The listing builds one solid part. Answer for the finished solid, in the listing's coordinates (mm). A direction names the side the tool comes from. Give positions to 0.01 mm unless a question says otherwise; leave off trailing zeros. Order: outer loops, then holes, each group sorted by start corner. A loop starts at its lowest first (then second) coordinate and runs counter-clockwise, first axis right, second up. Notation, with made-up numbers: (75.25, -15) -> (106.25, -15) arc R18 cw to (106.25, 17) -> close; hole circle Ø1 at (-18.5, 12). An arc over 180 degrees is marked (long way). Answer as a JSON object with one key per item and string values. Group by question number.
```python
from build123d import *

# Parameters (mm, degrees)
SKETCH1_W               = 88.9
SKETCH1_H               = 76.2
BOSS_EXTRUDE1_DEPTH     = 25.4
SKETCH2_R               = 4.1021
CUT_EXTRUDE1_DEPTH      = 19.05
SKETCH5_W               = 88.9
SKETCH5_H               = 0.127
BOSS_EXTRUDE2_DEPTH     = 50.8
SKETCH6_R               = 16.53116582
SKETCH6_R_2             = 8.0645
BOSS_EXTRUDE3_DEPTH     = 76.2
BOSS_EXTRUDE4_DEPTH     = 18.288
SKETCH8_W               = 50.8
SKETCH8_H               = 20.36233164
BOSS_EXTRUDE5_DEPTH     = 27.94
CUT_EXTRUDE6_REACH      = 168.187
CUT_EXTRUDE6_END_RADIUS = 8.0645
SKETCH13_W              = 6.477
SKETCH13_H              = 7.366
CUT_EXTRUDE7_DEPTH      = 22.9616
BOSS_EXTRUDE6_DEPTH     = 50.8
CUT_EXTRUDE8_REACH      = 168.129
SKETCH14_3_R            = 5.25
CUT_EXTRUDE9_DEPTH      = 9
CUT_EXTRUDE10_REACH     = 168.129
SKETCH16_W              = 50.8
SKETCH16_H              = 6.39233418
BOSS_EXTRUDE7_DEPTH     = 50.8
BOSS_EXTRUDE9_START     = 19.05
BOSS_EXTRUDE9_DEPTH     = 19.05
SKETCH22_W              = 7.366
SKETCH22_H              = 12.954
CUT_EXTRUDE15_DEPTH     = 28.4988
MIRROR5_START           = 19.05
MIRROR5_COPY_1_DEPTH    = 19.05
MIRROR5_COPY_2_SKETCH_W = 7.366
MIRROR5_COPY_2_SKETCH_H = 12.954
MIRROR5_COPY_2_DEPTH    = 28.4988
SKETCH25_R              = 5.125
BOSS_EXTRUDE10_DEPTH    = 6.35


with BuildPart() as part:
    # Sketch1 → Boss-Extrude1 (new body)
    with BuildSketch(Plane(origin=(0, 0, 0), x_dir=(0, 0, -1), z_dir=(1, 0, 0))):
        with Locations((44.45, 38.1)):
            Rectangle(SKETCH1_W, SKETCH1_H)
    extrude(amount=BOSS_EXTRUDE1_DEPTH)

    # Sketch2 → Cut-Extrude1 (cut)
    with BuildSketch(Plane.ZY):
        with Locations((-85.09, 19.05)):
            Circle(SKETCH2_R)
        with Locations((-3.81, 57.15)):
            Circle(SKETCH2_R)
        with Locations((-3.81, 19.05)):
            Circle(SKETCH2_R)
        with Locations((-85.09, 57.15)):
            Circle(SKETCH2_R)
    extrude(amount=-CUT_EXTRUDE1_DEPTH, mode=Mode.SUBTRACT)

    # Sketch5 → Boss-Extrude2 (add)
    with BuildSketch(Plane(origin=(25.4, 0, 0), x_dir=(0, 0, -1), z_dir=(1, 0, 0))):
        with Locations((44.45, 0.0635)):
            Rectangle(SKETCH5_W, SKETCH5_H)
    extrude(amount=BOSS_EXTRUDE2_DEPTH)

    # Sketch6 → Boss-Extrude3 (add)
    # profile 1 of 2: a face of its own
    with BuildSketch(Plane(origin=(25.4, 0, 0), x_dir=(0, 0, -1), z_dir=(1, 0, 0))):
        with Locations(Location((-1.7145, 38.1635, 0), (0, 0, 275.953033203))):
            Circle(SKETCH6_R)
        with Locations(Location((-1.7145, 38.1635, 0), (0, 0, 77.725329785))):
            Circle(SKETCH6_R_2, mode=Mode.SUBTRACT)
    # profile 2 of 2: a face of its own
    with BuildSketch(Plane(origin=(25.4, 0, 0), x_dir=(0, 0, -1), z_dir=(1, 0, 0))):
        with Locations(Location((90.6145, 38.1635, 0), (0, 0, 264.046966797))):
            Circle(SKETCH6_R)
        with Locations(Location((90.6145, 38.1635, 0), (0, 0, 102.274670215))):
            Circle(SKETCH6_R_2, mode=Mode.SUBTRACT)
    extrude(amount=BOSS_EXTRUDE3_DEPTH)

    # Sketch7 → Boss-Extrude4 (add)
    with BuildSketch(Plane.XY):
        Polygon((76.2, 0.127), (25.4, 0.127), (25.4, 76.2), (0, 76.2), (0, 58.670238274), (19.05, 58.670238274), (19.05, 55.629761726), (0, 55.629761726), (0, 20.570238274), (19.05, 20.570238274), (19.05, 17.529761726), (0, 17.529761726), (0, 0), (76.2, 0), align=None)
    boss_extrude4 = extrude(amount=BOSS_EXTRUDE4_DEPTH)

    # Mirror2: Boss-Extrude4 across plane
    add(boss_extrude4.mirror(Plane.XY.offset(-44.45)))

    # Sketch8 → Boss-Extrude5 (add)
    with BuildSketch(Plane(origin=(0, 0.127, 0), x_dir=(1, 0, 0), z_dir=(0, 1, 0))):
        with Locations((50.8, -1.7145)):
            Rectangle(SKETCH8_W, SKETCH8_H)
    boss_extrude5 = extrude(amount=BOSS_EXTRUDE5_DEPTH)

    # Cut-Extrude6: up to this cylinder (the profile starts outside it)
    cut_extrude6_end = Plane(origin=(57.15, 38.1635, 1.7145), z_dir=(-1, 0, 0)) * Cylinder(CUT_EXTRUDE6_END_RADIUS, 353.503, mode=Mode.PRIVATE)
    # Sketch12 → Cut-Extrude6 (cut, up to the surface)
    with BuildSketch(Plane.XZ, mode=Mode.PRIVATE) as cut_extrude6_sk1:
        with BuildLine():
            ThreePointArc((52.6669, 1.7145), (57.15, -2.7686), (61.6331, 1.7145))
            Line((61.6331, 1.7145), (52.6669, 1.7145))
        make_face()
    cut_extrude6_tool1 = extrude(cut_extrude6_sk1.sketch, amount=-CUT_EXTRUDE6_REACH, mode=Mode.PRIVATE) - cut_extrude6_end
    # Sketch12 → Cut-Extrude6 (cut, up to the surface)
    with BuildSketch(Plane.XZ, mode=Mode.PRIVATE) as cut_extrude6_sk2:
        with BuildLine():
            Line((52.6669, 1.7145), (61.6331, 1.7145))
            ThreePointArc((61.6331, 1.7145), (57.15, 6.1976), (52.6669, 1.7145))
        make_face()
    cut_extrude6_tool2 = extrude(cut_extrude6_sk2.sketch, amount=-CUT_EXTRUDE6_REACH, mode=Mode.PRIVATE) - cut_extrude6_end
    # Sketch12 → Cut-Extrude6 (cut, up to the surface)
    with BuildSketch(Plane.XZ, mode=Mode.PRIVATE) as cut_extrude6_sk3:
        with BuildLine():
            ThreePointArc((52.6669, 1.7145), (57.15, -2.7686), (61.6331, 1.7145))
            Line((61.6331, 1.7145), (52.6669, 1.7145))
        make_face()
    cut_extrude6_tool3 = extrude(cut_extrude6_sk3.sketch, amount=-CUT_EXTRUDE6_REACH, mode=Mode.PRIVATE) - cut_extrude6_end
    # Sketch12 → Cut-Extrude6 (cut, up to the surface)
    with BuildSketch(Plane.XZ, mode=Mode.PRIVATE) as cut_extrude6_sk4:
        with BuildLine():
            Line((52.6669, 1.7145), (61.6331, 1.7145))
            ThreePointArc((61.6331, 1.7145), (57.15, 6.1976), (52.6669, 1.7145))
        make_face()
    cut_extrude6_tool4 = extrude(cut_extrude6_sk4.sketch, amount=-CUT_EXTRUDE6_REACH, mode=Mode.PRIVATE) - cut_extrude6_end
    cut_extrude6 = cut_extrude6_tool1.solids().sort_by_distance((57.15, 0, -0.188187))[0] + cut_extrude6_tool2.solids().sort_by_distance((57.15, 0, 3.617187))[0] + cut_extrude6_tool3.solids().sort_by_distance((57.15, 0, -0.188187))[0] + cut_extrude6_tool4.solids().sort_by_distance((57.15, 0, 3.617187))[0]
    add(cut_extrude6, mode=Mode.SUBTRACT)

    # Sketch13 → Cut-Extrude7 (cut)
    with BuildSketch(Plane.XY.offset(18.288)):
        with Locations((60.3885, 17.94933418)):
            Rectangle(SKETCH13_W, SKETCH13_H)
        with Locations((53.9115, 17.94933418)):
            Rectangle(SKETCH13_W, SKETCH13_H)
    cut_extrude7 = extrude(amount=-CUT_EXTRUDE7_DEPTH, mode=Mode.SUBTRACT)

    # Mirror3: Boss-Extrude5, Cut-Extrude6, Cut-Extrude7 across plane
    add(boss_extrude5.mirror(Plane.XY.offset(-44.45)))
    add(cut_extrude6.mirror(Plane.XY.offset(-44.45)), mode=Mode.SUBTRACT)
    add(cut_extrude7.mirror(Plane.XY.offset(-44.45)), mode=Mode.SUBTRACT)

    # Sketch14 → Boss-Extrude6 (add)
    with BuildSketch(Plane(origin=(0, 0.127, 0), x_dir=(1, 0, 0), z_dir=(0, 1, 0))):
        Polygon((48.563230368, 37.763351356), (48.563230368, 51.136648644), (36.981615184, 57.823297288), (25.4, 51.136648644), (25.4, 37.763351356), (36.981615184, 31.076702712), align=None)
        Polygon((28.481615184, 49.357477288), (28.481615184, 39.542522712), (36.981615184, 34.635045424), (45.481615184, 39.542522712), (45.481615184, 49.357477288), (36.981615184, 54.264954576), align=None, mode=Mode.SUBTRACT)
    extrude(amount=BOSS_EXTRUDE6_DEPTH)

    # Sketch14<3> → Cut-Extrude8 (cut, up to next)
    with BuildSketch(Plane(origin=(0, 0.127, 0), x_dir=(1, 0, 0), z_dir=(0, 1, 0)), mode=Mode.PRIVATE) as cut_extrude8_sk1:
        with Locations(Location((36.981615184, 44.45, 0), (0, 0, 270))):
            Circle(SKETCH14_3_R)
    cut_extrude8_tool1 = extrude(cut_extrude8_sk1.sketch, amount=-CUT_EXTRUDE8_REACH, mode=Mode.PRIVATE) & part.part
    add(cut_extrude8_tool1.solids().sort_by_distance((36.981615, 0.127, -44.45))[0], mode=Mode.SUBTRACT)

    # Sketch15 → Cut-Extrude9 (cut)
    with BuildSketch(Plane.XZ):
        Polygon((45.531615184, -39.513655198), (36.981615184, -34.577310397), (28.431615184, -39.513655198), (28.431615184, -49.386344802), (36.981615184, -54.322689603), (45.531615184, -49.386344802), align=None)
    extrude(amount=-CUT_EXTRUDE9_DEPTH, mode=Mode.SUBTRACT)

    # Sketch16 → Cut-Extrude10 (cut, up to next)
    with BuildSketch(Plane(origin=(0, 0.127, 0), x_dir=(1, 0, 0), z_dir=(0, 1, 0)), mode=Mode.PRIVATE) as cut_extrude10_sk1:
        Polygon((48.563230368, 37.763351356), (36.981615184, 31.076702712), (25.4, 31.076702712), (25.4, 8.46666582), (76.2, 8.46666582), (76.2, 80.43333418), (25.4, 80.43333418), (25.4, 57.823297288), (36.981615184, 57.823297288), (48.563230368, 51.136648644), align=None)
    cut_extrude10_tool1 = extrude(cut_extrude10_sk1.sketch, amount=-CUT_EXTRUDE10_REACH, mode=Mode.PRIVATE) & part.part
    # Sketch16 → Cut-Extrude10 (cut, up to next)
    with BuildSketch(Plane(origin=(0, 0.127, 0), x_dir=(1, 0, 0), z_dir=(0, 1, 0)), mode=Mode.PRIVATE) as cut_extrude10_sk2:
        with Locations((50.8, -15.09183291)):
            Rectangle(SKETCH16_W, SKETCH16_H)
    cut_extrude10_tool2 = extrude(cut_extrude10_sk2.sketch, amount=-CUT_EXTRUDE10_REACH, mode=Mode.PRIVATE) & part.part
    # Sketch16 → Cut-Extrude10 (cut, up to next)
    with BuildSketch(Plane(origin=(0, 0.127, 0), x_dir=(1, 0, 0), z_dir=(0, 1, 0)), mode=Mode.PRIVATE) as cut_extrude10_sk3:
        with Locations((50.8, 103.99183291)):
            Rectangle(SKETCH16_W, SKETCH16_H)
    cut_extrude10_tool3 = extrude(cut_extrude10_sk3.sketch, amount=-CUT_EXTRUDE10_REACH, mode=Mode.PRIVATE) & part.part
    add(cut_extrude10_tool1.solids().sort_by_distance((53.397723, 0.127, -44.45))[0], mode=Mode.SUBTRACT)
    add(cut_extrude10_tool2.solids().sort_by_distance((50.8, 0.127, 15.091833))[0], mode=Mode.SUBTRACT)
    add(cut_extrude10_tool3.solids().sort_by_distance((50.8, 0.127, -103.991833))[0], mode=Mode.SUBTRACT)

    # Sketch18 → Boss-Extrude7 (add)
    with BuildSketch(Plane(origin=(0, 0.127, 0), x_dir=(1, 0, 0), z_dir=(0, 1, 0))):
        Polygon((36.981615184, 57.823297288), (25.4, 57.823297288), (25.4, 51.136648644), align=None)
        Polygon((25.4, 37.763351356), (25.4, 31.076702712), (36.981615184, 31.076702712), align=None)
    extrude(amount=BOSS_EXTRUDE7_DEPTH)

    # Sketch20 → Boss-Extrude9 (add)
    with BuildSketch(Plane.ZY.offset(-19.05).offset(BOSS_EXTRUDE9_START)):
        with BuildLine():
            ThreePointArc((0.2921, 19.05), (0.218413175, 18.275976935), (0, 17.529761726))
            Line((0, 17.529761726), (18.288, 17.529761726))
            Line((18.288, 17.529761726), (18.288, 20.570238274))
            Line((18.288, 20.570238274), (0, 20.570238274))
            ThreePointArc((0, 20.570238274), (0.218413175, 19.824023065), (0.2921, 19.05))
        make_face()
    boss_extrude9 = extrude(amount=-BOSS_EXTRUDE9_DEPTH)

    # Sketch22 → Cut-Extrude15 (cut)
    with BuildSketch(Plane.XY.offset(18.288)):
        with Locations((12.1412, 19.05)):
            Rectangle(SKETCH22_W, SKETCH22_H)
    cut_extrude15 = extrude(amount=-CUT_EXTRUDE15_DEPTH, mode=Mode.SUBTRACT)

    # Mirror4: Boss-Extrude9, Cut-Extrude15 across plane
    add(boss_extrude9.mirror(Plane.XY.offset(-44.45)))
    add(cut_extrude15.mirror(Plane.XY.offset(-44.45)), mode=Mode.SUBTRACT)

    # Mirror5: Boss-Extrude9, Cut-Extrude15 across plane
    add(boss_extrude9.mirror(Plane.ZX.offset(38.1)))
    add(cut_extrude15.mirror(Plane.ZX.offset(38.1)), mode=Mode.SUBTRACT)

    # Mirror5 copy 1 sketch → Mirror5 copy 1 (add)
    with BuildSketch(Plane(origin=(19.05, 76.2, -88.9), x_dir=(0, 0, -1), z_dir=(-1, 0, 0)).offset(MIRROR5_START)):
        with BuildLine():
            ThreePointArc((0.2921, 19.05), (0.218413175, 18.275976935), (0, 17.529761726))
            Line((0, 17.529761726), (18.288, 17.529761726))
            Line((18.288, 17.529761726), (18.288, 20.570238274))
            Line((18.288, 20.570238274), (0, 20.570238274))
            ThreePointArc((0, 20.570238274), (0.218413175, 19.824023065), (0.2921, 19.05))
        make_face()
    extrude(amount=-MIRROR5_COPY_1_DEPTH)

    # Mirror5 copy 2 sketch → Mirror5 copy 2 (cut)
    with BuildSketch(Plane(origin=(0, 76.2, -107.188), x_dir=(1, 0, 0), z_dir=(0, 0, -1))):
        with Locations((12.1412, 19.05)):
            Rectangle(MIRROR5_COPY_2_SKETCH_W, MIRROR5_COPY_2_SKETCH_H)
    extrude(amount=-MIRROR5_COPY_2_DEPTH, mode=Mode.SUBTRACT)

    # Sketch25 → Boss-Extrude10 (add)
    with BuildSketch(Plane(origin=(0, 9.000000034, 0), x_dir=(-1, 0, 0), z_dir=(0, -1, 0))):
        Polygon((-36.981615184, 34.577310397), (-28.431615184, 39.513655198), (-28.431615184, 49.386344802), (-36.981615184, 54.322689603), (-45.531615184, 49.386344802), (-45.531615184, 39.513655198), align=None)
        with Locations(Location((-36.981615184, 44.45, 0), (0, 0, 90))):
            Circle(SKETCH25_R, mode=Mode.SUBTRACT)
    extrude(amount=-BOSS_EXTRUDE10_DEPTH)


solid = part.part
```
(1) A cutting plane is placed at C-C (x = 39). Determine the outline of the cut face in (y, z).
(2) Find the intervals of material crossed by line 1 along Z through (x, y) = (3, 19.05); line 2 along X through (y, z) = (16, -96); line 3 along Y through (x, z) = (3, -85), in increasing order. Write a range as [from, to].
(3) Flat-ended cylindrical pins translate along their axes: pin 1 Ø1.5 at (y, z) = (58.5, -45) entering from +X; pin 2 Ø4 at (y, z) = (56.5, -87) entering from -X; pin 3 Ø3 at (x, y) = (90.5, 35.5) entering from +Z; pin 4 Ø4 at (y, z) = (55, -5.5) entering from -X. Find the tip coordinate at first contact, or state that the pin passes through.
(4) A cutting plane is placed at A-A (x = 57.15). State how many separate pieces and enclosed holes the cut face has, and give its area (3 significant figures).
(5) For a pull along Z with two mould halves and no side action, classify faces 5 (the flat face through (15.824, 19, 4)), 6 (the flat face through (12, 57, -10.211)), 7 (the cylindrical face through (53.01, 26.48, -92.33)), 8 (the flat face through (13, 39, -107.188)) as +Z half, -Z half, draft (parallel to the pull), parting line (faces both ways), or undercut.
(6) Which of the six approach directions +Z, -Z, +X, -X, +Y, -Y give full straight-line access (tool end or side, diameter ignored) to faces 1 (the flat face through (41.291, 32.889, -51.777)), 2 (the flat face through (19.05, 57, -4)), 3 (the flat face through (63.627, 18, 4)), 4 (the flat face through (12, 63.627, -93))?
(7) A cutting plane is placed at B-B (z = -44.45). Determine the outline of the cut face in (x, y).
Check sheet entries:
{
 "1": {"outline": "(0, -100.8) -> (25.14, -100.8) arc R16.53 ccw (long way) to (25.14, -80.43) -> (0, -80.43) -> close; (0, -56.66) -> (50.93, -56.66) -> (50.93, -53.1) -> (15.35, -53.1) -> (15.35, -49.16) -> (9, -49.16) -> (9, -53.16) -> (0, -53.16) -> close; (0, -35.74) -> (9, -35.74) -> (9, -39.74) -> (15.35, -39.74) -> (15.35, -35.8) -> (50.93, -35.8) -> (50.93, -32.24) -> (0, -32.24) -> close; (0, -8.47) -> (25.14, -8.47) arc R16.53 ccw (long way) to (25.14, 11.9) -> (0, 11.9) -> close; hole circle Ø16.13 at (38.16, -90.61); hole circle Ø16.13 at (38.16, 1.71)"},
 "2": {"line 1": "z = [-107.19, -89.19], [-80.99, -7.91], [0.29, 18.29]", "line 2": "x = [0, 8.46], [15.82, 50.67], [63.63, 76.2]", "line 3": "y = [0, 14.95], [23.15, 53.05], [61.25, 76.2]"},
 "3": {"pin 1": "stops at x = 25.4", "pin 2": "stops at x = 19.05", "pin 3": "stops at z = 18.2", "pin 4": "stops at x = 0"},
 "4": {"separate pieces": "4", "enclosed holes": "0", "area": "1,580 mm2"},
 "5": {"face 5": "draft", "face 6": "+Z half", "face 7": "undercut", "face 8": "-Z half"},
 "6": {"face 1": "+Y", "face 2": "-X", "face 3": "+Z", "face 4": "-Z"},
 "7": {"outline": "(0, 0) -> (28.43, 0) -> (28.43, 9) -> (31.86, 9) -> (31.86, 15.35) -> (28.48, 15.35) -> (28.48, 50.93) -> (25.4, 50.93) -> (25.4, 76.2) -> (0, 76.2) -> close; (42.11, 9) -> (45.53, 9) -> (45.53, 0) -> (48.56, 0) -> (48.56, 50.93) -> (45.48, 50.93) -> (45.48, 15.35) -> (42.11, 15.35) -> close"}
}
